from build123d import *

# Parameters (mm, degrees)
BOSS_EXTRUDE2_DEPTH = 2
CHAMFER2_SIZE       = 12
FILLET1_R           = 7.5
SKETCH2_R           = 2.575
SKETCH2_R_2         = 3
CUT_EXTRUDE1_DEPTH  = 290.359637821


with BuildPart() as part:
    # Sketch1 → Boss-Extrude2 (new body)
    with BuildSketch(Plane(origin=(0, 0, 0), x_dir=(1, 0, 0), z_dir=(0, 1, 0))):
        Polygon((40, -50), (77.320508076, -40), (285, -40), (285, 40), (77.320508076, 40), (40, 50), (-40, 50), (-157, 50), (-157, -50), (-40, -50), align=None)
    extrude(amount=BOSS_EXTRUDE2_DEPTH)

    # Chamfer2
    chamfer2_edges = [part.edges().sort_by_distance(p)[0] for p in [
        (-157, 1, 50),
        (-157, 1, -50),
        (285, 1, -40),
        (285, 1, 40),
    ]]
    chamfer(chamfer2_edges, length=CHAMFER2_SIZE)

    # Fillet1
    fillet1_edges = [part.edges().sort_by_distance(p)[0] for p in [
        (40, 1, -50),
        (77.320508076, 1, -40),
        (77.320508076, 1, 40),
        (40, 1, 50),
        (-145, 1, 50),
        (-157, 1, -38),
        (-157, 1, 38),
        (-145, 1, -50),
        (273, 1, -40),
        (285, 1, 28),
        (285, 1, -28),
        (273, 1, 40),
    ]]
    fillet(fillet1_edges, radius=FILLET1_R)

    # Sketch2 → Cut-Extrude1 (cut, through all)
    with BuildSketch(Plane(origin=(0, 2, 0), x_dir=(1, 0, 0), z_dir=(0, 1, 0))):
        with Locations(Location((-40, 40, 0), (0, 0, 270))):
            Circle(SKETCH2_R)
        with Locations(Location((40, 40, 0), (0, 0, 90))):
            Circle(SKETCH2_R)
        with Locations(Location((40, -40, 0), (0, 0, 270))):
            Circle(SKETCH2_R)
        with Locations(Location((-40, -40, 0), (0, 0, 90))):
            Circle(SKETCH2_R)
        with Locations(Location((0, 0, 0), (0, 0, 270))):
            Circle(SKETCH2_R_2)
    extrude(amount=-CUT_EXTRUDE1_DEPTH, mode=Mode.SUBTRACT)


solid = part.part
Design review of the part built by this model. Coordinates are the model's own, in mm. Give positions to 0.01 mm unless a question says otherwise; leave off trailing zeros. Loops run counter-clockwise (first coordinate to the right, second up) from the corner with the lowest first, then second, coordinate; pieces in that order, holes last. Notation, with made-up numbers: (39.25, -18.5) -> (59.25, -18.5) arc R17 cw to (59.25, -14.5) -> close; hole circle Ø7 at (33.5, 49). An arc over 180 degrees is marked (long way). One line per question, with ' | ' between items. Start each with the question number.
(1) Insertion check: P1, Ø5.5, axis at x = 0, z = 0, coming from the +Y side; P2, Ø6.5, axis at x = -40, z = -40, coming from the -Y side. Each pin has a flat end and moves straight along its axis. Give the tip position at first contact, or say it passes through.
(2) We need section A-A (y = 0.8). State how many separate pieces and enclosed holes the cut face has, and give its area (3 significant figures).
(3) We need section B-B (x = 112). State the section outline as (y, z) points.
(4) Draft analysis for pull direction X (two halves, no side actions). For faces 1 (the face through (279, 1, 34)), 2 (the face through (61, 0, -1)), 3 (the face through (-151, 1, -44)), state which applies: +X half, -X half, draft (parallel to the pull), parting line (faces both ways), or undercut.
(5) For line 1 (Z direction, x = -41, y = 1.2); line 2 (Z direction, x = 119, y = 1.65); line 3 (X direction, y = 1.25, z = 28.5), list the stretches that pass through material, from the lowest coordinate up.
The answers:
1) P1: passes through | P2: stops at y = 0
2) separate pieces: 1 | enclosed holes: 5 | area: 39,300 mm^2
3) outline: (0, -40) -> (2, -40) -> (2, 40) -> (0, 40) -> close
4) face 1: +X half | face 2: draft | face 3: -X half
5) line 1: z = -50 to -42.37, -37.63 to 37.63, 42.37 to 50 | line 2: z = -40 to 40 | line 3: x = -157 to 284.08
